Autodesk Inventor part; units mm, degrees
ref_plane "Work Plane1" through (0, 0, 9.525) normal (0, 0, 1) x (1, 0, 0)
ref_plane "YZ Plane" through (0, 0, 0) normal (1, 0, 0) x (0, 1, 0)
ref_plane "XZ Plane" through (0, 0, 0) normal (0, 1, 0) x (-1, 0, 0)
sketch "Sketch1" plane through (0, 0, 0) normal (0, 0, 1) x (1, 0, 0)
  line L0 (0, 9.525) -> (0, -9.525)
  arc A0 (0, -9.525) -> (0, 9.525) centre (0, 0) ccw
  dimension "d0" = 9.525
revolve "Revolution1" add sketch "Sketch1" angle 360 about axis through (0, 9.525, 0) along (0, -1, 0)
ref_plane "Work Plane1" through (0, 0, 9.525) normal (0, 0, 1) x (1, 0, 0)
sketch "Sketch2" plane through (0, 0, 9.525) normal (0, 0, 1) x (1, 0, 0)
  circle A0 centre (0, 0) radius 3.9751
  dimension "d2" = 7.9502
extrude "Extrusion1" cut sketch "Sketch2" against normal blind 12.7
sketch "Sketch3" plane through (0, 0, 0) normal (0, 1, 0) x (-1, 0, 0)
  circle A0 centre (0, 0) radius 1.3208
  dimension "d5" = 2.6416
extrude "Extrusion2" cut sketch "Sketch3" along normal through all both and the other way through all
properties part number "Handle_Ball" material "Steel, Mild"
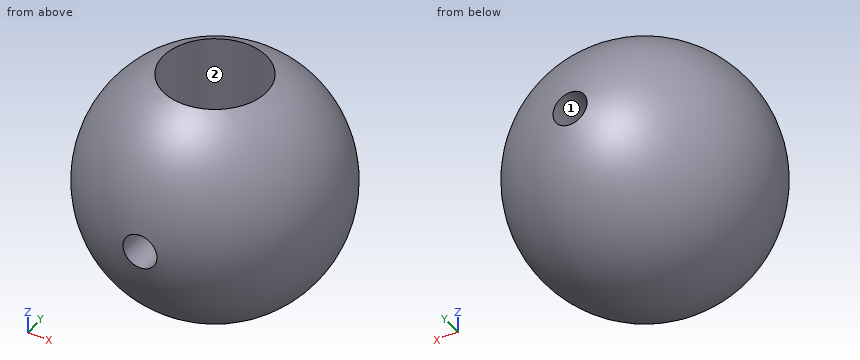
CAD build for the part. Positions are in the model's coordinates, mm. Face numbers are marked on the shaded views. A direction names the side the tool comes from. Round coordinates to 2 decimals unless told otherwise and drop trailing zeros. Loops run counter-clockwise (first coordinate to the right, second up) from the corner with the lowest first, then second, coordinate; pieces in that order, holes last.
(1) Cut at A-A (z = 0). Give the cut face in (x, y) (3 decimals), plus the area to 3 significant figures.
(2) Which spindle directions (+Z, -Z, +X, -X, +Y, -Y) get a long thin tool onto all of the face, cutting with end or side? Do the marked faces 1 and 2. Say none if no direction does.
(3) Cut at C-C (y = 0). Give the cut face in (x, z) (3 decimals), plus the area to 3 significant figures.
(4) Cut at B-B (x = 0). Give the cut face in (y, z) (3 decimals), plus the area to 3 significant figures.
(5) Cut at D-D (y = -7.75). Give the cut face in (x, z).
(6) Wall check: line 1 along Y through (x, z) = (-1, -1); line 2 along Y through (x, z) = (-2.5, 2); line 3 along Z through (x, y) = (0, -5.25). Give the ranges that are in metal, low to high.
(7) Drop flat-ended pins along their axis: pin 1 (8 mm diameter, centred on y = -5.5, z = 5, fed in from +X); pin 2 (1 mm diameter, centred on x = 7.5, z = 3.5, fed in from -Y); pin 3 (4 mm diameter, centred on y = 7, z = -1, fed in from +X); pin 4 (2.5 mm diameter, centred on x = 0, z = 0, fed in from -Y). Give the stop position or say it passes through.
Findings below:
1. outline: (-1.321, -9.433) - (-1.321, -3.749) arc R3.975 cw to (-1.321, 3.749) - (-1.321, 9.433) arc R9.525 ccw to start; (1.321, -9.433) arc R9.525 ccw to (1.321, 9.433) - (1.321, 3.749) arc R3.975 cw to (1.321, -3.749) - close
1. area: 206 mm2
2. face 1: +Y, -Y
2. face 2: +Z
3. outline: (-3.975, -3.175) - (-3.975, 8.656) arc R9.525 ccw (long way) to (3.975, 8.656) - (3.975, -3.175) - close
3. area: 186 mm2
4. outline: (-9.433, -1.321) arc R9.525 ccw to (9.433, -1.321) - (3.975, -1.321) - (3.975, -3.175) - (-3.975, -3.175) - (-3.975, -1.321) - close; (-9.433, 1.321) - (-3.975, 1.321) - (-3.975, 8.656) arc R9.525 ccw to start; (3.975, 1.321) - (9.433, 1.321) arc R9.525 ccw to (3.975, 8.656) - close
4. area: 157 mm2
5. outline: circle Ø11.07 at (0, 0); hole circle Ø2.64 at (0, 0)
6. line 1: y = -9.42 to -3.85, 3.85 to 9.42
6. line 2: y = -8.97 to -3.09, 3.09 to 8.97
6. line 3: z = -7.95 to -1.32, 1.32 to 7.95
7. pin 1: stops at x = 8.88
7. pin 2: stops at y = -5.5
7. pin 3: stops at x = 8.06
7. pin 4: passes through
